from build123d import *

# Parameters (mm, degrees)
F0_R      = 42.25
F1_DEPTH  = 11
F2_R      = 42.25
F2_R_2    = 40.75
F3_DEPTH  = 5
F4_R      = 39.88
F5_DEPTH  = 6
F6_R      = 2.5
F6_R_2    = 4
F7_DEPTH  = 5.001
F8_R      = 19.05
F9_DEPTH  = 1.6
F10_R     = 22.5
F11_DEPTH = 49
F12_R     = 15.5
F13_DEPTH = 52.401
F14_R     = 17.5
F14_R_2   = 15.5
F15_DEPTH = 14.6
F17_R     = 18.9
F18_DEPTH = 1.6
F19_SIZE  = 1
F20_R     = 4.5
F21_DEPTH = 42.251


with BuildPart() as f1:
    # F0 (on Front) → F1 (new body)
    with BuildSketch(Plane.XZ):
        Circle(F0_R)
    extrude(amount=F1_DEPTH)

    # F2 (on face) → F3 (cut)
    with BuildSketch(Plane.XZ.offset(11)):
        Circle(F2_R)
        Circle(F2_R_2, mode=Mode.SUBTRACT)
    extrude(amount=-F3_DEPTH, mode=Mode.SUBTRACT)

    # F4 (on face) → F5 (cut)
    with BuildSketch(Plane.XZ.offset(11)):
        Circle(F4_R)
    extrude(amount=-F5_DEPTH, mode=Mode.SUBTRACT)

    # F6 (on face) → F7 (cut, through all)
    with BuildSketch(Plane.XZ.offset(5)):
        with Locations((-23.57, 23.57)):
            Circle(F6_R)
        with Locations((23.57, 23.57)):
            Circle(F6_R)
        with Locations((23.57, -23.57)):
            Circle(F6_R)
        with Locations((-23.57, -23.57)):
            Circle(F6_R)
        with Locations((0, 35)):
            Circle(F6_R_2)
    extrude(amount=-F7_DEPTH, mode=Mode.SUBTRACT)

    # F8 (on face) → F9 (cut)
    with BuildSketch(Plane.XZ.offset(5)):
        Circle(F8_R)
    extrude(amount=-F9_DEPTH, mode=Mode.SUBTRACT)

    # F10 (on face) → F11 (join)
    with BuildSketch(Plane(origin=(0, 0, 0), x_dir=(-1, 0, 0), z_dir=(0, 1, 0))):
        Circle(F10_R)
    extrude(amount=F11_DEPTH)

    # F12 (on face) → F13 (cut, through all)
    with BuildSketch(Plane.XZ.offset(3.4)):
        Circle(F12_R)
    extrude(amount=-F13_DEPTH, mode=Mode.SUBTRACT)

    # F14 (on face) → F15 (cut)
    with BuildSketch(Plane(origin=(0, 49, 0), x_dir=(-1, 0, 0), z_dir=(0, 1, 0))):
        Circle(F14_R)
        Circle(F14_R_2, mode=Mode.SUBTRACT)
    extrude(amount=-F15_DEPTH, mode=Mode.SUBTRACT)

    # F17 (on offset) → F18 (cut)
    with BuildSketch(Plane(origin=(0, 46, 0), x_dir=(-1, 0, 0), z_dir=(0, 1, 0))):
        Circle(F17_R)
    extrude(amount=-F18_DEPTH, mode=Mode.SUBTRACT)

    # F19
    f19_edges = [f1.edges().sort_by_distance(p)[0] for p in [
        (22.5, 49, 0),
        (17.5, 49, 0),
        (-42.25, 0, 0),
        (-42.25, -6, 0),
    ]]
    chamfer(f19_edges, length=F19_SIZE)

    # F20 (on Top) → F21 (cut, through all)
    with BuildSketch(Plane.XY):
        with Locations((0, 5.5)):
            Circle(F20_R)
    extrude(amount=-F21_DEPTH, mode=Mode.SUBTRACT)


solid = f1.part
Can you work these out from the model? Positions are in its coordinate system, mm. A direction names the side the tool comes from. Give positions to 0.01 mm unless a question says otherwise; leave off trailing zeros. Loops run counter-clockwise (first coordinate to the right, second up) from the corner with the lowest first, then second, coordinate; pieces in that order, holes last. Notation, with made-up numbers: M -0.75,-11 L 21.25,-11 A22 ccw 21.25,12 Z; hole C 69.25,50.25 d11. An arc over 180 degrees is marked long. One line per item, written item: value. Start each with the question number.
1) I'm going to push flat-ended pins straight in: pin 1 (19 mm diameter, centred on x = -6.5, z = -9, fed in from -Y); pin 2 (3 mm diameter, centred on x = -18, z = 27.5, fed in from +Y); pin 3 (14.5 mm diameter, centred on x = 0, y = 5.5, fed in from -Z). Where does each tip first touch, or does it pass through?
2) On a 3-axis mill with a long thin cutter (end or side, diameter ignored), from which of +Z, -Z, +X, -X, +Y, -Y can I reach the whole of each face in a straight line? I mean faces 4 (the face through (-10.382, 23.664, -19.961)), 5 (the face through (-15.12, -4.21, -11.59)), 6 (the face through (-17, 46, -6)). Say none if no direction works.
3) If we section it at D-D, the plane y = 14: Write out the boundary of the cut face in (x, z), and give its area (3 significant figures).
4) If I drill on line 1 (Z direction, x = 0, y = -4); line 2 (Z direction, x = 0, y = -8); line 3 (Z direction, x = 0, y = 32), over which ranges is the centre line in solid material (lowest first)? Write a range as [from, to].
5) If we section it at B-B, the plane z = 23.57: Give the number of separate pieces and of enclosed holes in the cut face, and give its area (3 significant figures).
6) If we section it at A-A, the plane y = 37: Write out the boundary of the cut face in (x, z), and give its area (3 significant figures).
7) Thinking about a two-plate mould opening in Y: for faces 1 (the face through (13.887, 39.47, -10.648)), 2 (the face through (-18.027, 45.211, 5.677)), 3 (the face through (18, 0, -18)), which applies, +Y half, -Y half, draft (parallel to the pull), parting line (faces both ways), or undercut?
Completed:
1. pin 1: stops at y = -5
1. pin 2: stops at y = 0
1. pin 3: stops at z = -42.25
2. face 4: +Y
2. face 5: -Y
2. face 6: none
3. outline: C 0,0 d45; hole C 0,0 d31
3. area: 836 mm^2
4. line 1: z = [-42.25, -19.05], [19.05, 31], [39, 42.25]
4. line 2: z = [-40.75, -39.88], [39.88, 40.75]
4. line 3: z = [-22.5, -15.5], [15.5, 22.5]
5. separate pieces: 3
5. enclosed holes: 0
5. area: 315 mm^2
6. outline: C 0,0 d45; hole C 0,0 d35
6. area: 628 mm^2
7. face 1: draft
7. face 2: undercut
7. face 3: +Y half
